```python
from build123d import *

# Parameters (mm, degrees)
SKETCH_1_W      = 20
SKETCH_1_H      = 8
EXTRUDE_1_DEPTH = 12
SKETCH_5_W      = 8
SKETCH_5_H      = 8
EXTRUDE_5_DEPTH = 10
SKETCH_8_W      = 20
SKETCH_8_H      = 8
EXTRUDE_6_DEPTH = 55
SKETCH_9_W      = 12
SKETCH_9_H      = 8
EXTRUDE_7_DEPTH = 15
SKETCH_10_W     = 12
SKETCH_10_H     = 8
EXTRUDE_8_DEPTH = 15


with BuildPart() as part:
    # ｽｹｯﾁ1 → ﾎﾞｽ - 押し出し1 (new body)
    with BuildSketch(Plane.XY):
        Rectangle(SKETCH_1_W, SKETCH_1_H)
    extrude(amount=EXTRUDE_1_DEPTH)

    # ｽｹｯﾁ5 → ﾎﾞｽ - 押し出し5 (add)
    with BuildSketch(Plane(origin=(0, 0, 0), x_dir=(-1, 0, 0), z_dir=(0, 0, -1))):
        Rectangle(SKETCH_5_W, SKETCH_5_H)
    extrude(amount=EXTRUDE_5_DEPTH)

    # ｽｹｯﾁ8 → ﾎﾞｽ - 押し出し6 (add)
    with BuildSketch(Plane.XY.offset(12)):
        Rectangle(SKETCH_8_W, SKETCH_8_H)
    extrude(amount=EXTRUDE_6_DEPTH)

    # ｽｹｯﾁ9 → ﾎﾞｽ - 押し出し7 (add)
    with BuildSketch(Plane(origin=(10, 0, 0), x_dir=(0, 0, -1), z_dir=(1, 0, 0))):
        with Locations((-6, 0)):
            Rectangle(SKETCH_9_W, SKETCH_9_H)
    extrude(amount=EXTRUDE_7_DEPTH)

    # ｽｹｯﾁ10 → ﾎﾞｽ - 押し出し8 (add)
    with BuildSketch(Plane.ZY.offset(10)):
        with Locations((6, 0)):
            Rectangle(SKETCH_10_W, SKETCH_10_H)
    extrude(amount=EXTRUDE_8_DEPTH)


solid = part.part
```
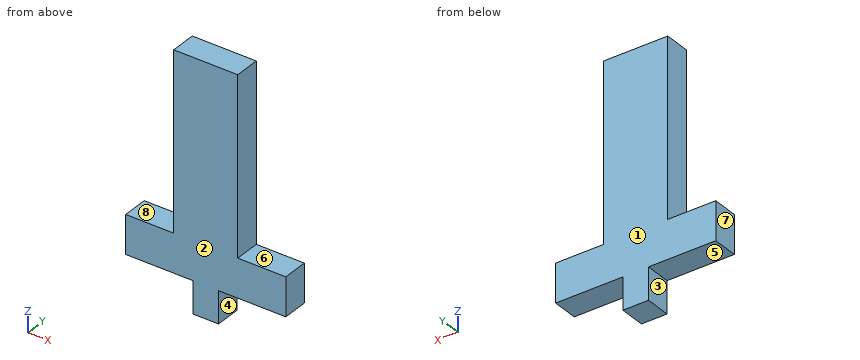
Verification items for the finished model (mm, model axes). Face numbers are marked on the shaded views. A direction names the side the tool comes from. Give positions to 0.01 mm unless a question says otherwise; leave off trailing zeros. Order: outer loops, then holes, each group sorted by start corner. A loop starts at its lowest first (then second) coordinate and runs counter-clockwise, first axis right, second up. Notation, with made-up numbers: M 32,70.25 L 70,70.25 A16 ccw 70,97.25 Z; hole C 54,10 d8. An arc over 180 degrees is marked long. Return JSON: item names as keys, results as strings. Group by question number.
1) Go/stop test with flat-tipped pins: pin 1 Ø1.5 at (x, y) = (-12.5, 0.5) entering from -Z; pin 2 Ø4 at (y, z) = (-1.5, -4) entering from +X; pin 3 Ø2.5 at (x, y) = (18, 1) entering from +Z; pin 4 Ø6 at (x, z) = (13.5, 44.5) entering from -Y. Record where each tip stops, or that it passes through.
2) Access from +Z, -Z, +X, -X, +Y, -Y to the whole of each face (thin tool, end or side, straight path). Record for the marked faces 4, 5, 6, 7 and 8.
3) Section check B-B on z = 53. Record the cut outline in (x, y).
4) Scan lines: line 1 (Z direction, x = 11, y = -0.25); line 2 (Z direction, x = -9.5, y = 0); line 3 (X direction, y = -1.25, z = 46.5). Record each from-to range of solid material in increasing order.
5) Mould release check, pull along Y, two halves, no side actions. Record for the marked faces 1, 2 and 3: pulls with the +Y half, pulls with the -Y half, needs draft (parallel to the pull), parting line crosses it, or undercut.
6) Section check C-C on x = -7. Record the cut outline in (y, z), and give its area (3 significant figures).
7) Section check A-A on y = 2.5. Record the cut outline in (x, z), and give its area (3 significant figures).
Answer block:
{
 "1": {"pin 1": "stops at z = 0", "pin 2": "stops at x = 4", "pin 3": "stops at z = 12", "pin 4": "passes through"},
 "2": {"face 4": "-Z, +X, +Y, -Y", "face 5": "-Z, -X, +Y, -Y", "face 6": "+Z, +X, +Y, -Y", "face 7": "+Z, -Z, -X, +Y, -Y", "face 8": "+Z, -X, +Y, -Y"},
 "3": {"outline": "M -10,-4 L 10,-4 L 10,4 L -10,4 Z"},
 "4": {"line 1": "z = 0 to 12", "line 2": "z = 0 to 67", "line 3": "x = -10 to 10"},
 "5": {"face 1": "pulls with the +Y half", "face 2": "pulls with the -Y half", "face 3": "needs draft"},
 "6": {"outline": "M -4,0 L 4,0 L 4,67 L -4,67 Z", "area": "536 mm^2"},
 "7": {"outline": "M -25,0 L -4,0 L -4,-10 L 4,-10 L 4,0 L 25,0 L 25,12 L 10,12 L 10,67 L -10,67 L -10,12 L -25,12 Z", "area": "1,780 mm^2"}
}
